For this review, take the finished solid that the model builds, in its own axes (mm). Round coordinates to 2 decimals unless told otherwise and drop trailing zeros. Write each loop counter-clockwise with the first axis right and the second up, starting at its lowest first coordinate (ties: lowest second). Pieces come first, ordered by that corner, then holes. Notation, with made-up numbers: M 1,-33.75 L 5,-33.75 A10 cw 5,-15.75 Z; hole C 82.25,39 d1. An arc over 180 degrees is marked long. Answer in a Markdown table with one row per item.
```python
from build123d import *

# Parameters (mm, degrees)
SKETCH_1_R      = 1.75
SKETCH_1_R_2    = 2
EXTRUDE_1_DEPTH = 1.5


with BuildPart() as part:
    # Эскиз1 → Бобышка-Вытянуть1 (new body)
    with BuildSketch(Plane(origin=(0, 0, 0), x_dir=(1, 0, 0), z_dir=(0, 1, 0))):
        with BuildLine():
            Line((208.5, 12.5), (208.5, 22))
            Line((208.5, 22), (0, 22))
            Line((0, 22), (0, 0))
            Line((0, 0), (286.5, 0))
            Line((286.5, 0), (286.5, 16))
            Line((286.5, 16), (277.5, 16))
            Line((277.5, 16), (277.5, 12.5))
            ThreePointArc((277.5, 12.5), (276.621320344, 10.378679656), (274.5, 9.5))
            Line((274.5, 9.5), (211.5, 9.5))
            ThreePointArc((211.5, 9.5), (209.378679656, 10.378679656), (208.5, 12.5))
        make_face()
        with Locations((206.5, 7.5)):
            Circle(SKETCH_1_R, mode=Mode.SUBTRACT)
        with Locations((279.5, 7.5)):
            Circle(SKETCH_1_R_2, mode=Mode.SUBTRACT)
        with Locations((15, 16)):
            Circle(SKETCH_1_R, mode=Mode.SUBTRACT)
        with Locations((71, 16)):
            Circle(SKETCH_1_R, mode=Mode.SUBTRACT)
        with Locations((128, 16)):
            Circle(SKETCH_1_R, mode=Mode.SUBTRACT)
        with Locations((184, 16)):
            Circle(SKETCH_1_R, mode=Mode.SUBTRACT)
    extrude(amount=EXTRUDE_1_DEPTH)


solid = part.part
```
Q1. For probe 1 along Z at (x, y) = (15, 1.1); probe 2 along X at (y, z) = (0.1, -12.25); probe 3 along X at (y, z) = (0.4, -16.5), list the stretches that pass through material, from the lowest coordinate up.
Found:
| item | result |
|---|---|
| probe 1 | -22 to -17.75, -14.25 to 0 |
| probe 2 | 0 to 208.51, 277.49 to 286.5 |
| probe 3 | 0 to 13.32, 16.68 to 69.32, 72.68 to 126.32, 129.68 to 182.32, 185.68 to 208.5 |
Q2. Take a section at A-A (y = 0.3). State the section outline as (x, z) points.
Found:
| item | result |
|---|---|
| outline | M 0,-22 L 208.5,-22 L 208.5,-12.5 A3 cw 211.5,-9.5 L 274.5,-9.5 A3 cw 277.5,-12.5 L 277.5,-16 L 286.5,-16 L 286.5,0 L 0,0 Z; hole C 15,-16 d3.5; hole C 71,-16 d3.5; hole C 128,-16 d3.5; hole C 184,-16 d3.5; hole C 206.5,-7.5 d3.5; hole C 279.5,-7.5 d4 |
Q3. Insertion check: P1, Ø0.8, axis at x = 247, y = 1, coming from the -Z side. The pin has a flat end and moves straight along its axis. Give the tip position at first contact, or say it passes through.
Found:
| item | result |
|---|---|
| P1 | z = -9.5 |
